Could you check a few things on this model? Use its own coordinates, in mm. Face numbers are marked on the shaded views. A direction names the side the tool comes from. Give positions to 0.01 mm unless a question says otherwise; leave off trailing zeros. Loops run counter-clockwise (first coordinate to the right, second up) from the corner with the lowest first, then second, coordinate; pieces in that order, holes last. Notation, with made-up numbers: M -25,29.5 L 8,29.5 A18 cw 8,37.5 Z; hole C -10,52 d1. An arc over 180 degrees is marked long. Return JSON: item names as keys, results as strings. Group by question number.
1. If we section it at C-C (y = 6): Write out the boundary of the cut face in (x, z).
2. If we section it at A-A (z = 0): State how many separate pieces and enclosed holes the cut face has, plus the area to 3 significant figures.
3. Please list where these lines run through material, in increasing order: line 1 (Z direction, x = 19.5, y = 0.45); line 2 (Z direction, x = -7, y = 4.5); line 3 (Y direction, x = 20, z = -2).
4. If we section it at D-D (x = 19.5): Write out the boundary of the cut face in (y, z).
5. For pin 1 (1.5 mm diameter, centred on x = 10, y = 9.5, fed in from +Z); pin 2 (12 mm diameter, centred on y = 15, z = -8, fed in from -X); pin 3 (1.5 mm diameter, centred on y = 8, z = 4, fed in from -X), each with a flat end and sliding along its axis, tell me the tip position at first contact or that it passes through.
6. If we section it at B-B (x = -18): Write out the boundary of the cut face in (y, z), plus the area to 3 significant figures.
7. For the marked faces 1 and 2, which set-ups out of +Z, -Z, +X, -X, +Y, -Y let a thin tool reach every point of the face, with its end or its side?
```python
from build123d import *

# Parameters (mm, degrees)
SKETCH1_R           = 2
BOSS_EXTRUDE1_DEPTH = 1


with BuildPart() as part:
    # Sketch1 → Boss-Extrude1 (new body)
    with BuildSketch(Plane(origin=(0, 0, 0), x_dir=(1, 0, 0), z_dir=(0, 1, 0))):
        with BuildLine():
            Line((-23.414655011, 2.20086192), (-9.740182864, 12.693653445))
            ThreePointArc((-9.740182864, 12.693653445), (0, 16), (9.740182864, 12.693653445))
            Line((9.740182864, 12.693653445), (23.414655011, 2.20086192))
            ThreePointArc((23.414655011, 2.20086192), (24.5, 0), (23.414655011, -2.20086192))
            Line((23.414655011, -2.20086192), (9.740182864, -12.693653445))
            ThreePointArc((9.740182864, -12.693653445), (0, -16), (-9.740182864, -12.693653445))
            Line((-9.740182864, -12.693653445), (-23.414655011, -2.20086192))
            ThreePointArc((-23.414655011, -2.20086192), (-24.5, 0), (-23.414655011, 2.20086192))
        make_face()
        with Locations(Location((-19.5, 0, 0), (0, 0, 270))):
            Circle(SKETCH1_R, mode=Mode.SUBTRACT)
        with Locations(Location((19.5, 0, 0), (0, 0, 90))):
            Circle(SKETCH1_R, mode=Mode.SUBTRACT)
    extrude(amount=BOSS_EXTRUDE1_DEPTH)

    # Sketch2 → Revolve1 (revolve)
    with BuildSketch(Plane.XY, mode=Mode.PRIVATE) as revolve1_sk:
        with BuildLine():
            Line((0, 6.082034509), (0, 1))
            Line((0, 1), (-14.5, 1))
            Line((-14.5, 1), (-14.5, 7.345083381))
            ThreePointArc((-14.5, 7.345083381), (-12.078795143, 14.399662879), (-5.835769403, 18.480588566))
            ThreePointArc((-5.835769403, 18.480588566), (-3.178192824, 20.343251845), (0, 21))
            Line((0, 21), (0, 6.082034509))
        make_face()
    revolve(revolve1_sk.sketch.rotate(Axis((0, 0, 0), (0, 1, 0)), 270), axis=Axis((0, 0, 0), (0, 1, 0)))


solid = part.part
```
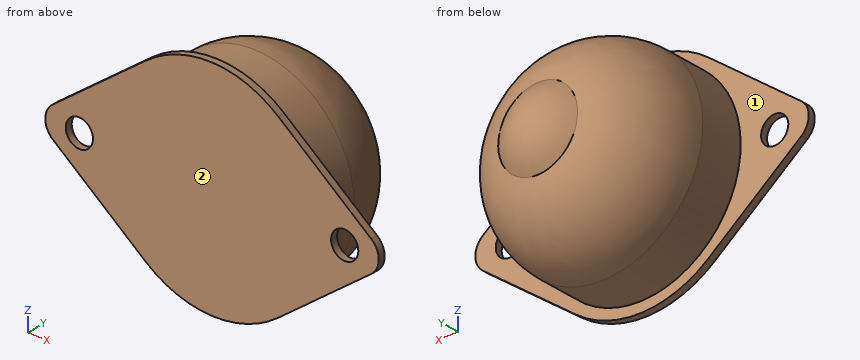
Answer:
{
 "1": {"outline": "C 0,0 d29"},
 "2": {"separate pieces": "3", "enclosed holes": "0", "area": "518 mm²"},
 "3": {"line 1": "z = -5.2 to -2, 2 to 5.2", "line 2": "z = -12.7 to 12.7", "line 3": "y = 0 to 1"},
 "4": {"outline": "M 0,-5.2 L 1,-5.2 L 1,-2 L 0,-2 Z; M 0,2 L 1,2 L 1,5.2 L 0,5.2 Z"},
 "5": {"pin 1": "stops at z = 10.92", "pin 2": "stops at x = -13.47", "pin 3": "stops at x = -14.12"},
 "6": {"outline": "M 0,-6.36 L 1,-6.36 L 1,-1.32 L 0,-1.32 Z; M 0,1.32 L 1,1.32 L 1,6.36 L 0,6.36 Z", "area": "10.1 mm²"},
 "7": {"face 1": "+Y", "face 2": "+Z, -Z, +X, -X, -Y"}
}
